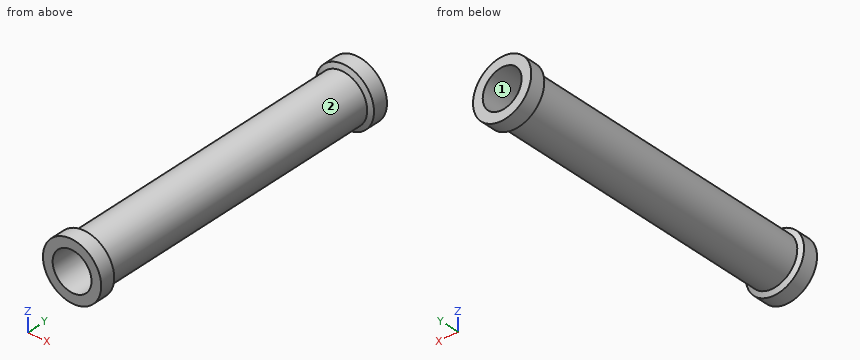
```python
from build123d import *

# Parameters (mm, degrees)
F0_R     = 19.05
F0_R_2   = 12.7
F1_DEPTH = 152.4
F2_DEPTH = 57.15


with BuildPart() as f1:
    # F0 (on Front) → F1 (new body)
    with BuildSketch(Plane.XZ):
        Circle(F0_R)
        Circle(F0_R_2, mode=Mode.SUBTRACT)
    extrude(amount=F1_DEPTH)

    # F2 (add): a face of the model
    f2_faces = [f1.faces().sort_by_distance(p)[0] for p in [
        (-18.5111846327, -152.4, 0),
    ]]
    extrude(f2_faces, amount=F2_DEPTH)

    # F3 (on Right) → F4 (revolve, cut)
    with BuildSketch(Plane.YZ):
        Polygon((-11.023053821, 15.9428958603), (-6.3529792242, 25.6566461176), (-203.1970207758, 25.6566461176), (-198.526946179, 15.9428958603), align=None)
    revolve(axis=Axis((0, -209.55, 0), (0, -1, 0)), mode=Mode.SUBTRACT)


solid = f1.part
```
Verification items for the finished model (mm, model axes). Face numbers are marked on the shaded views. Round coordinates to 2 decimals unless told otherwise and drop trailing zeros. Order: outer loops, then holes, each group sorted by start corner. A loop starts at its lowest first (then second) coordinate and runs counter-clockwise, first axis right, second up. Notation, with made-up numbers: (62, 44.25) - (118, 44.25) arc R30 ccw to (118, 75.25) - close; hole circle Ø11 at (71.5, 84.25). An arc over 180 degrees is marked (long way). Use CSV: the item, a comma, the result in double quotes. Start each with the question number.
1) Go/stop test with flat-tipped pins: P1, Ø1.5, axis at x = -15, z = -14.5, coming from the +Y side; P2, Ø8, axis at x = -14, y = -123.5, coming from the -Z side; P3, Ø4, axis at x = -11.5, y = -23.5, coming from the +Z side; P4, Ø12, axis at x = -4, z = -9, coming from the -Y side. Record where each tip stops, or that it passes through.
2) Section check B-B, the plane x = 0. Record the cut outline in (y, z), plus the area to 3 significant figures.
3) Mould release check, pull along Z, two halves, no side actions. Record for the marked faces 1 and 2: +Z half, -Z half, draft (parallel to the pull), parting line (faces both ways), or undercut.
4) Thickness scan on L1, parallel to Z at x = 0, y = -42; L2, parallel to X at y = -183, z = 4; L3, parallel to X at y = -23, z = -4.5. Record the ranges inside material, lowest first.
5) Section check C-C, the plane y = -18. Record the cut outline in (x, z).
6) Section check A-A, the plane z = 0. Record the cut outline in (x, y).
Answers:
1,P1,"passes through"
1,P2,"stops at z = -12.42"
1,P3,"stops at z = 12.8"
1,P4,"stops at y = -209.55"
2,outline,"(-209.55, -19.05) - (-200.02, -19.05) - (-198.53, -15.94) - (-11.02, -15.94) - (-9.53, -19.05) - (0, -19.05) - (0, -12.7) - (-209.55, -12.7) - close; (-209.55, 12.7) - (0, 12.7) - (0, 19.05) - (-9.53, 19.05) - (-11.02, 15.94) - (-198.53, 15.94) - (-200.02, 19.05) - (-209.55, 19.05) - close"
2,area,"1,490 mm²"
3,face 1,"undercut"
3,face 2,"parting line"
4,L1,"z = -15.94 to -12.7, 12.7 to 15.94"
4,L2,"x = -15.43 to -12.05, 12.05 to 15.43"
4,L3,"x = -15.29 to -11.88, 11.88 to 15.29"
5,outline,"circle Ø31.89 at (0, 0); hole circle Ø25.4 at (0, 0)"
6,outline,"(-19.05, -209.55) - (-12.7, -209.55) - (-12.7, 0) - (-19.05, 0) - (-19.05, -9.53) - (-15.94, -11.02) - (-15.94, -198.53) - (-19.05, -200.02) - close; (12.7, -209.55) - (19.05, -209.55) - (19.05, -200.02) - (15.94, -198.53) - (15.94, -11.02) - (19.05, -9.53) - (19.05, 0) - (12.7, 0) - close"
